Design review of the part built by this model. Coordinates are the model's own, in mm. Coordinates: 2 decimals unless noted, no trailing zeros. Loops run counter-clockwise (first coordinate to the right, second up) from the corner with the lowest first, then second, coordinate; pieces in that order, holes last. Notation, with made-up numbers: (24.25, -17.5) - (51.25, -17.5) arc R31 cw to (51.25, 7.5) - close; hole circle Ø1 at (40, 18.5). An arc over 180 degrees is marked (long way). Answer in a Markdown table with one row per item. Add a question column.
(1) We need section B-B, the plane x = 15.5. Write out the cut boundary in (y, z), plus the area to 3 significant figures.
(2) Clearance check with flat-ended pins moving along their axes: pin 1 (1.8 mm diameter, centred on x = 15, y = 21, fed in from -Z); pin 2 (1.5 mm diameter, centred on y = 2.5, z = -5.5, fed in from -X); pin 3 (10 mm diameter, centred on y = 3.5, z = -5.5, fed in from +X). State where each tip first meets the part, or that it passes through.
(3) We need section C-C, the plane y = 8. Write out the cut boundary in (x, z).
(4) We need section D-D, the plane z = 1.5. Write out the cut boundary in (x, y), plus the area to 3 significant figures.
(5) To check wall thickness, follow L1, parallel to Y at x = 15.5, z = 1.15; L2, parallel to Z at x = 27.5, y = 6.5; L3, parallel to Y at x = 28.5, z = -6.5. State the ranges of each line that lie inside material, in increasing order. Write a range as [from, to].
(6) We need section A-A, the plane y = 20. Write out the cut boundary in (x, z).
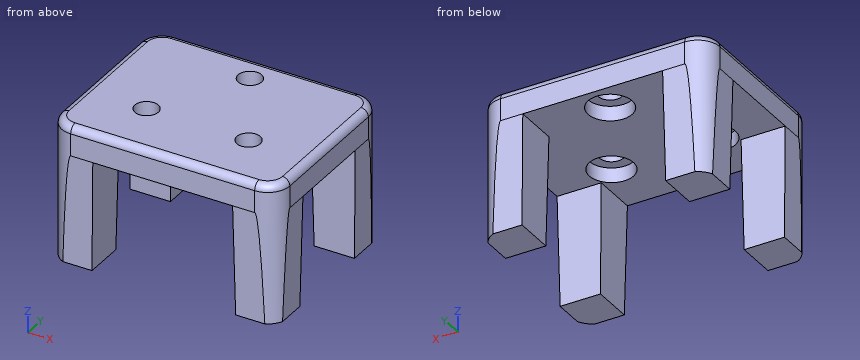
from build123d import *

# Parameters (mm, degrees)
SKETCH1_W                     = 6
SKETCH1_H                     = 6
BOSS_EXTRUDE1_DEPTH           = 4
SKETCH1_3_W                   = 6
SKETCH1_3_H                   = 6
BOSS_EXTRUDE2_DEPTH           = 15
BOSS_EXTRUDE2_DRAFT           = -1
BOSS_EXTRUDE2_PROFILE_2_DEPTH = 15
BOSS_EXTRUDE2_PROFILE_2_DRAFT = -1
BOSS_EXTRUDE2_PROFILE_3_DEPTH = 15
BOSS_EXTRUDE2_PROFILE_3_DRAFT = -1
BOSS_EXTRUDE2_PROFILE_4_DEPTH = 15
BOSS_EXTRUDE2_PROFILE_4_DRAFT = -1
SKETCH2_R                     = 1.6
CUT_EXTRUDE1_DEPTH            = 42.976183724
SKETCH3_R                     = 3
CUT_EXTRUDE2_DEPTH            = 2
FILLET1_R                     = 3
FILLET2_R                     = 1


with BuildPart() as part:
    # Sketch1 → Boss-Extrude1 (new body)
    with BuildSketch(Plane.XY):
        Polygon((6, 6), (6, 0), (25, 0), (25, 6), (31, 6), (31, 18), (25, 18), (25, 24), (6, 24), (6, 18), (0, 18), (0, 6), align=None)
        with Locations((3, 21)):
            Rectangle(SKETCH1_W, SKETCH1_H)
        with Locations((3, 3)):
            Rectangle(SKETCH1_W, SKETCH1_H)
        with Locations((28, 21)):
            Rectangle(SKETCH1_W, SKETCH1_H)
        with Locations((28, 3)):
            Rectangle(SKETCH1_W, SKETCH1_H)
    extrude(amount=BOSS_EXTRUDE1_DEPTH)


with BuildPart() as boss_extrude2_tool:
    # Sketch1<3> → Boss-Extrude2 (with draft: the straight prism first)
    with BuildSketch(Plane.XY):
        with Locations((3, 21)):
            Rectangle(SKETCH1_3_W, SKETCH1_3_H)
    extrude(amount=-BOSS_EXTRUDE2_DEPTH)
    # Boss-Extrude2: the draft: its side faces are tilted about the plane it starts from
    boss_extrude2_sides = [boss_extrude2_tool.faces().sort_by_distance(p)[0] for p in [
        (3, 24, -7.5),
        (0, 21, -7.5),
        (3, 18, -7.5),
        (6, 21, -7.5),
    ]]
    draft(boss_extrude2_sides, Plane.XY, BOSS_EXTRUDE2_DRAFT)


with BuildPart() as part_1:
    add(part.part)

    # Boss-Extrude2: add boss_extrude2_tool
    add(boss_extrude2_tool.part)


with BuildPart() as boss_extrude2_profile_2_tool:
    # Sketch1<3> → Boss-Extrude2 profile 2 (with draft: the straight prism first)
    with BuildSketch(Plane.XY):
        with Locations((28, 21)):
            Rectangle(SKETCH1_3_W, SKETCH1_3_H)
    extrude(amount=-BOSS_EXTRUDE2_PROFILE_2_DEPTH)
    # Boss-Extrude2 profile 2: the draft: its side faces are tilted about the plane it starts from
    boss_extrude2_profile_2_sides = [boss_extrude2_profile_2_tool.faces().sort_by_distance(p)[0] for p in [
        (28, 18, -7.5),
        (31, 21, -7.5),
        (28, 24, -7.5),
        (25, 21, -7.5),
    ]]
    draft(boss_extrude2_profile_2_sides, Plane.XY, BOSS_EXTRUDE2_PROFILE_2_DRAFT)


with BuildPart() as part_2:
    add(part_1.part)

    # Boss-Extrude2 profile 2: add boss_extrude2_profile_2_tool
    add(boss_extrude2_profile_2_tool.part)


with BuildPart() as boss_extrude2_profile_3_tool:
    # Sketch1<3> → Boss-Extrude2 profile 3 (with draft: the straight prism first)
    with BuildSketch(Plane.XY):
        with Locations((28, 3)):
            Rectangle(SKETCH1_3_W, SKETCH1_3_H)
    extrude(amount=-BOSS_EXTRUDE2_PROFILE_3_DEPTH)
    # Boss-Extrude2 profile 3: the draft: its side faces are tilted about the plane it starts from
    boss_extrude2_profile_3_sides = [boss_extrude2_profile_3_tool.faces().sort_by_distance(p)[0] for p in [
        (28, 0, -7.5),
        (31, 3, -7.5),
        (28, 6, -7.5),
        (25, 3, -7.5),
    ]]
    draft(boss_extrude2_profile_3_sides, Plane.XY, BOSS_EXTRUDE2_PROFILE_3_DRAFT)


with BuildPart() as part_3:
    add(part_2.part)

    # Boss-Extrude2 profile 3: add boss_extrude2_profile_3_tool
    add(boss_extrude2_profile_3_tool.part)


with BuildPart() as boss_extrude2_profile_4_tool:
    # Sketch1<3> → Boss-Extrude2 profile 4 (with draft: the straight prism first)
    with BuildSketch(Plane.XY):
        with Locations((3, 3)):
            Rectangle(SKETCH1_3_W, SKETCH1_3_H)
    extrude(amount=-BOSS_EXTRUDE2_PROFILE_4_DEPTH)
    # Boss-Extrude2 profile 4: the draft: its side faces are tilted about the plane it starts from
    boss_extrude2_profile_4_sides = [boss_extrude2_profile_4_tool.faces().sort_by_distance(p)[0] for p in [
        (0, 3, -7.5),
        (3, 0, -7.5),
        (6, 3, -7.5),
        (3, 6, -7.5),
    ]]
    draft(boss_extrude2_profile_4_sides, Plane.XY, BOSS_EXTRUDE2_PROFILE_4_DRAFT)


with BuildPart() as part_4:
    add(part_3.part)

    # Boss-Extrude2 profile 4: add boss_extrude2_profile_4_tool
    add(boss_extrude2_profile_4_tool.part)

    # Sketch2 → Cut-Extrude1 (cut, through all)
    with BuildSketch(Plane(origin=(0, 0, 0), x_dir=(-1, 0, 0), z_dir=(0, 0, -1))):
        with Locations((-22.42820323, 8)):
            Circle(SKETCH2_R)
        with Locations((-15.5, 20)):
            Circle(SKETCH2_R)
        with Locations((-8.57179677, 8)):
            Circle(SKETCH2_R)
    extrude(amount=-CUT_EXTRUDE1_DEPTH, mode=Mode.SUBTRACT)

    # Sketch3 → Cut-Extrude2 (cut)
    with BuildSketch(Plane(origin=(0, 0, 0), x_dir=(-1, 0, 0), z_dir=(0, 0, -1))):
        with Locations((-15.5, 20)):
            Circle(SKETCH3_R)
        with Locations((-8.57179677, 8)):
            Circle(SKETCH3_R)
        with Locations((-22.42820323, 8)):
            Circle(SKETCH3_R)
    extrude(amount=-CUT_EXTRUDE2_DEPTH, mode=Mode.SUBTRACT)

    # Fillet1
    # the kernel refuses this fillet: 3 mm, written as the material it takes off along each edge
    with BuildSketch(Plane(origin=(31, 24, -18), x_dir=(-1, 0, 0), z_dir=(0, 0, 1)), Plane(origin=(31, 0, -18), x_dir=(0, 1, 0), z_dir=(0, 0, 1))) as fillet1_piece_1:
        with BuildLine():
            CenterArc((FILLET1_R, FILLET1_R), FILLET1_R, 180, 90)
            Line((0, FILLET1_R), (-FILLET1_R * 0.02, FILLET1_R))
            Line((-FILLET1_R * 0.02, FILLET1_R), (-FILLET1_R * 0.02, -FILLET1_R * 0.02))
            Line((-FILLET1_R * 0.02, -FILLET1_R * 0.02), (FILLET1_R, -FILLET1_R * 0.02))
            Line((FILLET1_R, -FILLET1_R * 0.02), (FILLET1_R, 0))
        make_face()
    extrude(amount=40, mode=Mode.SUBTRACT)
    with BuildSketch(Plane(origin=(0, 0, -18), x_dir=(0, 1, 0), z_dir=(0, 0, 1)), Plane(origin=(0, 24, -18), x_dir=(1, 0, 0), z_dir=(0, 0, 1))) as fillet1_piece_2:
        with BuildLine():
            CenterArc((FILLET1_R, -FILLET1_R), FILLET1_R, 90, 90)
            Line((0, -FILLET1_R), (-FILLET1_R * 0.02, -FILLET1_R))
            Line((-FILLET1_R * 0.02, -FILLET1_R), (-FILLET1_R * 0.02, FILLET1_R * 0.02))
            Line((-FILLET1_R * 0.02, FILLET1_R * 0.02), (FILLET1_R, FILLET1_R * 0.02))
            Line((FILLET1_R, FILLET1_R * 0.02), (FILLET1_R, 0))
        make_face()
    extrude(amount=40, mode=Mode.SUBTRACT)

    # Fillet2
    fillet2_edges = [part_4.edges().sort_by_distance(p)[0] for p in [
        (15.5, 24, 4),
        (31, 12, 4),
        (0, 12, 4),
        (15.5, 0, 4),
        (0.878679656, 23.121320344, 4),
        (0.878679656, 0.878679656, 4),
        (30.121320344, 0.878679656, 4),
        (30.121320344, 23.121320344, 4),
    ]]
    fillet(fillet2_edges, radius=FILLET2_R)


solid = part_4.part
Responses:
| question | item | result |
|---|---|---|
| 1 | outline | (0, 0) - (17, 0) - (17, 2) - (18.4, 2) - (18.4, 4) - (1, 4) arc R1 ccw to (0, 3) - close; (21.6, 2) - (23, 2) - (23, 0) - (24, 0) - (24, 3) arc R1 ccw to (23, 4) - (21.6, 4) - close |
| 1 | area | 77.2 mm2 |
| 2 | pin 1 | stops at z = 2 |
| 2 | pin 2 | stops at x = 0.08 |
| 2 | pin 3 | stops at x = 30.99 |
| 3 | outline | (0, 0) - (5.57, 0) - (5.57, 2) - (6.97, 2) - (6.97, 4) - (1, 4) arc R1 ccw to (0, 3) - close; (10.17, 2) - (11.57, 2) - (11.57, 0) - (19.43, 0) - (19.43, 2) - (20.83, 2) - (20.83, 4) - (10.17, 4) - close; (24.03, 2) - (25.43, 2) - (25.43, 0) - (31, 0) - (31, 3) arc R1 ccw to (30, 4) - (24.03, 4) - close |
| 4 | outline | (0, 3) arc R3 ccw to (3, 0) - (28, 0) arc R3 ccw to (31, 3) - (31, 21) arc R3 ccw to (28, 24) - (3, 24) arc R3 ccw to (0, 21) - close; hole circle Ø6 at (8.57, 8); hole circle Ø6 at (15.5, 20); hole circle Ø6 at (22.43, 8) |
| 4 | area | 651 mm2 |
| 5 | L1 | y = [0, 17], [23, 24] |
| 5 | L2 | z = [0, 4] |
| 5 | L3 | y = [0.11, 5.89], [18.11, 23.89] |
| 6 | outline | (0, 0) - (0.26, -15) - (5.74, -15) - (6, 0) - (12.5, 0) - (12.5, 2) - (13.9, 2) - (13.9, 4) - (1, 4) arc R1 ccw to (0, 3) - close; (17.1, 2) - (18.5, 2) - (18.5, 0) - (25, 0) - (25.26, -15) - (30.74, -15) - (31, 0) - (31, 3) arc R1 ccw to (30, 4) - (17.1, 4) - close |
